Study the drawing (mm; zero at the part's minimum x, y, z) and answer. Give positions to 0.01 mm unless a question says otherwise; leave off trailing zeros. Loops run counter-clockwise (first coordinate to the right, second up) from the corner with the lowest first, then second, coordinate; pieces in that order, holes last. Notation, with made-up numbers: M 20.25,-15.5 L 46.25,-15.5 A21 cw 46.25,9.5 Z; hole C -32.5,67.5 d10. An arc over 180 degrees is marked long. Return JSON: item names as keys, results as strings.
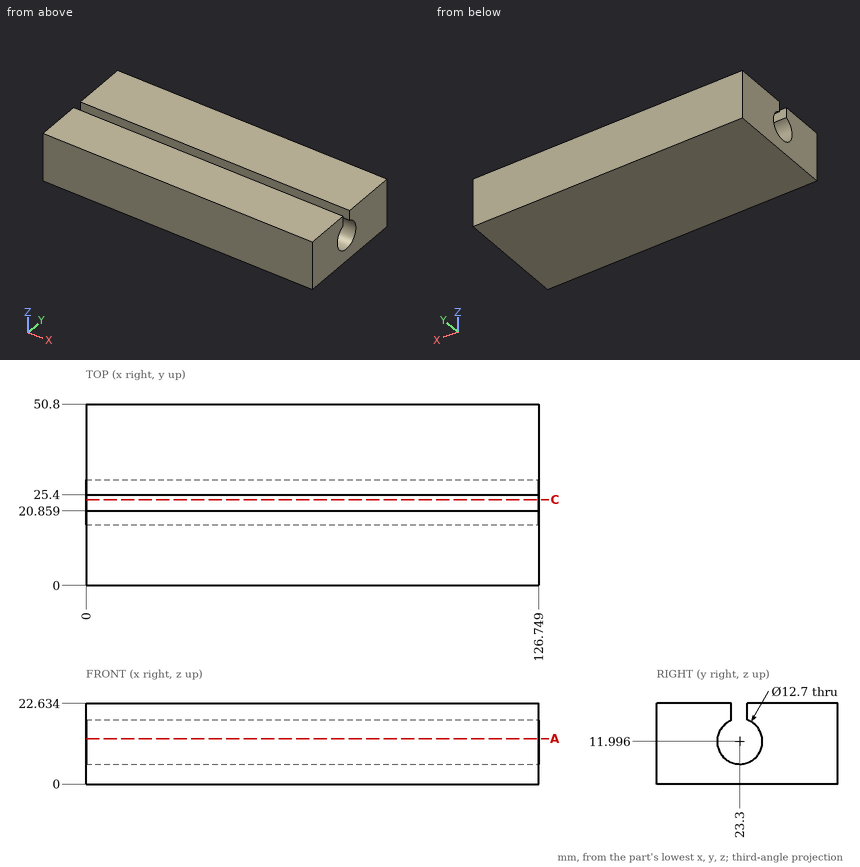
(1) The part is cut by section C-C (y = 24). Determine the outline of the cut face in (x, z) (1 decimal).
Values follow:
{"outline": "M 0,0 L 126.7,0 L 126.7,5.7 L 0,5.7 Z"}
(2) Straight lines are drawn through the part: line 1 along Y through (x, z) = (101, 20.5); line 2 along Z through (x, y) = (17, 27.5) (1 decimal); line 3 along Y through (x, z) = (52, 7.75). For each, find the intervals that lie inside material, in ascending order.
Values follow:
{"line 1": "0 to 20.86, 25.4 to 50.8", "line 2": "0 to 7.2, 16.8 to 22.6", "line 3": "0 to 18.58, 28.02 to 50.8"}
(3) The part is cut by section A-A (z = 12.75). Determine the outline of the cut face in (x, y) (1 decimal), and give its area (3 significant figures).
Values follow:
{"outline": "M 0,0 L 126.7,0 L 126.7,17 L 0,17 Z; M 0,29.6 L 126.7,29.6 L 126.7,50.8 L 0,50.8 Z", "area": "4,840 mm²"}
(4) Given pin 1 (3 mm diameter, centred on x = 102.5, y = 6.5, fed in from -Z), flat-ended and moving along its own axis, determine where the tip first touches the part or whether it passes through.
Values follow:
{"pin 1": "z = 0"}
